Input: dimensioned drawing with shaded views. Units: mm. Origin: part minimum x, y, z. Give positions to 0.01 mm unless a question says otherwise; leave off trailing zeros. Order: outer loops, then holes, each group sorted by start corner. A loop starts at its lowest first (then second) coordinate and runs counter-clockwise, first axis right, second up. Notation, with made-up numbers: (26, -15.5) - (62, -15.5) arc R15 ccw to (62, -2.5) - close; hole circle Ø4 at (-8.5, 87). An arc over 180 degrees is marked (long way). Answer as CSV lines item,"result".
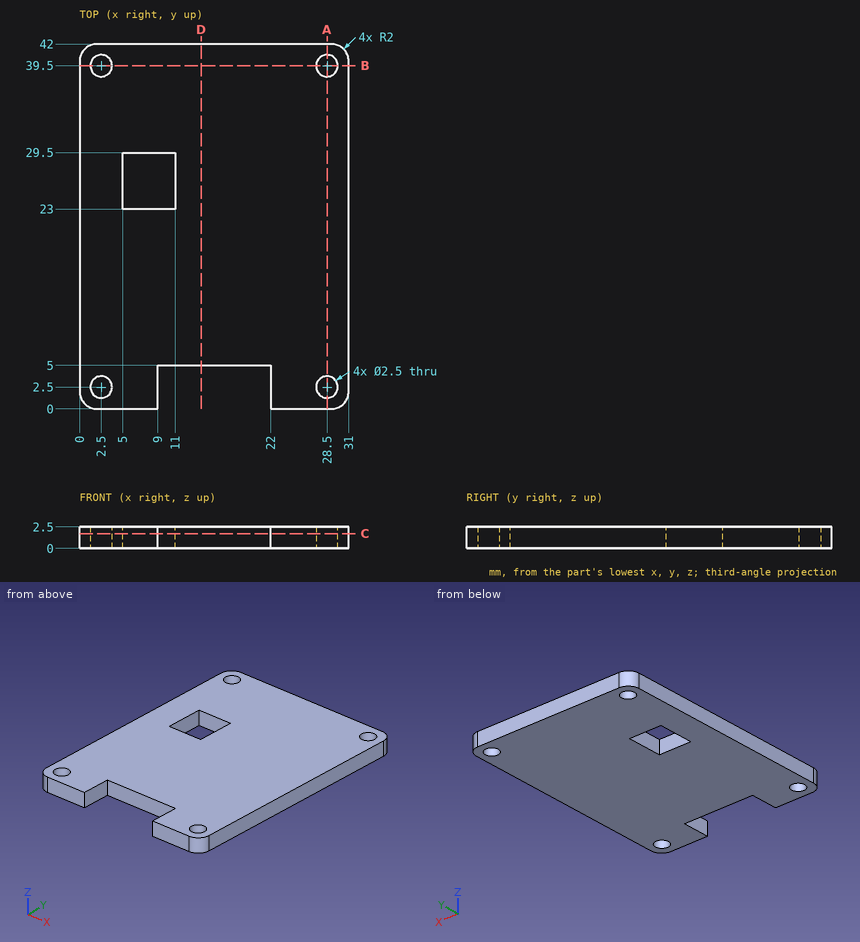
(1) Contact query for flat-ended pins moving along their axis: pin 1 (0.8 mm diameter, centred on x = 17.5, z = 1.5, fed in from -Y); pin 2 (1.2 mm diameter, centred on y = 26.5, z = 1.5, fed in from -X). Output: stop coordinate, or through.
Completed:
pin 1,"y = 5"
pin 2,"x = 0"
(2) Cut plane D-D (x = 14). Return loops of the section in (y, z), then the cut area to 3 significant figures.
Completed:
outline,"(5, 0) - (42, 0) - (42, 2.5) - (5, 2.5) - close"
area,"92.5 mm²"
(3) Cut plane C-C (z = 1.7). Return loops of the section in (x, y).
Completed:
outline,"(0, 2) arc R2 ccw to (2, 0) - (9, 0) - (9, 5) - (22, 5) - (22, 0) - (29, 0) arc R2 ccw to (31, 2) - (31, 40) arc R2 ccw to (29, 42) - (2, 42) arc R2 ccw to (0, 40) - close; hole circle Ø2.5 at (2.5, 2.5); hole circle Ø2.5 at (2.5, 39.5); hole (5, 23) - (11, 23) - (11, 29.5) - (5, 29.5) - close; hole circle Ø2.5 at (28.5, 2.5); hole circle Ø2.5 at (28.5, 39.5)"
(4) Cut plane B-B (y = 39.5). Return loops of the section in (x, z).
Completed:
outline,"(0, 0) - (1.25, 0) - (1.25, 2.5) - (0, 2.5) - close; (3.75, 0) - (27.25, 0) - (27.25, 2.5) - (3.75, 2.5) - close; (29.75, 0) - (31, 0) - (31, 2.5) - (29.75, 2.5) - close"
(5) Ray query, line 1 (X direction, y = 39.5, z = 0.75); line 2 (Y direction, x = 28.5, z = 0.6); line 3 (X direction, y = 4, z = 0.9). Return the intervals inside material, ascending. Write a range as from..to.
Completed:
line 1,"0..1.25, 3.75..27.25, 29.75..31"
line 2,"0..1.25, 3.75..38.25, 40.75..42"
line 3,"0..9, 22..31"
(6) Cut plane A-A (x = 28.5). Return loops of the section in (y, z), then the cut area to 3 significant figures.
Completed:
outline,"(0, 0) - (1.25, 0) - (1.25, 2.5) - (0, 2.5) - close; (3.75, 0) - (38.25, 0) - (38.25, 2.5) - (3.75, 2.5) - close; (40.75, 0) - (42, 0) - (42, 2.5) - (40.75, 2.5) - close"
area,"92.5 mm²"
